The listing builds one solid part. Answer for the finished solid, in the listing's coordinates (mm). A direction names the side the tool comes from. Coordinates: 2 decimals unless noted, no trailing zeros. Write each loop counter-clockwise with the first axis right and the second up, starting at its lowest first coordinate (ties: lowest second). Pieces come first, ordered by that corner, then holes.
(1) Given P1, Ø3.5, axis at x = -12, y = 0.5, coming from the +Z side; P2, Ø12, axis at x = -16, z = 6, coming from the +Y side; P3, Ø0.9, axis at x = -11, y = -1.5, coming from the +Z side; P4, Ø3, axis at x = -17, y = -2, coming from the +Z side, each flat-ended and moving along its own axis, determine where each tip first touches the part or whether it passes through.
(2) The part is cut by section B-B on y = -2.05. Determine the outline of the cut face in (x, z), plus the area to 3 significant figures.
(3) Which of the six approach directions +Z, -Z, +X, -X, +Y, -Y give full straight-line access (tool end or side, diameter ignored) to faces 4 (the flat face through (-13, 0, -10)), 5 (the flat face through (-10.495, -0.042, 11.702)), 6 (the flat face through (-10, 0, -13)), 7 (the cylindrical face through (-0.07, -0.04, -1.5))?
(4) Straight lines are drawn through the part: line 1 (X direction, y = 0.7, z = 0); line 2 (Z direction, x = -8.75, y = 0.3); line 3 (Z direction, x = -12.5, y = 0.7). For each, find the intervals that lie inside material, in ascending order.
(5) The part is cut by section C-C on z = -15. Determine the outline of the cut face in (x, y).
(6) The part is cut by section A-A on z = 0. Determine the outline of the cut face in (x, y), plus the area to 3 significant figures.
(7) For a pull along Z with two mould halves and no side action, classify faces 1 (the flat face through (-12, 0, -11.5)), 2 (the cylindrical face through (-19.43, -0.04, -20.4)), 3 (the cylindrical face through (4, 0, -3)) as +Z half, -Z half, draft (parallel to the pull), parting line (faces both ways), or undercut.
(8) The part is cut by section D-D on x = -2.5. Determine the outline of the cut face in (y, z).
Autodesk Inventor part; units mm, degrees
ref_plane "YZ Plane" through (0, 0, 0) normal (1, 0, 0) x (0, 1, 0)
ref_plane "XZ Plane" through (0, 0, 0) normal (0, 1, 0) x (-1, 0, 0)
ref_plane "XY Plane" through (0, 0, 0) normal (0, 0, 1) x (1, 0, 0)
sketch "Szkic1" plane through (0, 0, 0) normal (0, 1, 0) x (-1, 0, 0)
  arc A0 (13.307, 18.2188) -> (4.1253, 22.1807) centre (8.7161, 20.1997) ccw
  line L0 (4.1253, 22.1807) -> (-4.5909, 1.9809)
  line L1 (13.307, 18.2188) -> (7.6031, 5)
  arc A1 (-4.5909, 1.9809) -> (0, -5) centre (0, 0) ccw
  line L2 (8, -5) -> (10.5, -5) construction
  line L3 (10, -19) -> (10, -20)
  line L4 (10, -20) -> (10, -21)
  line L5 (10, -7) -> (10, -5)
  line L6 (10, -12) -> (10, -14)
  line L7 (10, -14) -> (10, -14.5)
  line L8 (20, -21) -> (10, -21)
  line L9 (13, -18) -> (10, -18)
  line L10 (10, -18) -> (10, -19)
  line L11 (10, -7) -> (10, -8)
  line L12 (10, -8) -> (13, -8)
  line L13 (13, -11.5) -> (10, -11.5)
  line L14 (10, -11.5) -> (10, -12)
  line L15 (13, -14.5) -> (10, -14.5)
  line L16 (10, -18) -> (13, -18)
  line L17 (13, -8) -> (13, -11.5)
  line L18 (13, -14.5) -> (13, -18)
  line L19 (18, 5) -> (20, 5)
  line L20 (20, 5) -> (20, -21)
  line L21 (20, -21) -> (18, -21)
  line L22 (0, -5) -> (10, -5)
  line L23 (18, 5) -> (7.6031, 5)
  arc A2 (13.307, 18.2188) -> (4.1253, 22.1807) centre (8.7161, 20.1997) ccw
extrude "Wyciągnięcie proste6" add sketch "Szkic1" along normal mid plane 6
fillet "Zaokrąglenie3" radius 2 2 edges at (-20, 0, -21) (-20, 0, 5)
fillet_without_effect "Fillet4"
sketch "Sketch8" plane through (0, 3, 0) normal (0, 1, 0) x (1, 0, 0)
  point P0 (0, 0)
  point P1 (0, 0)
hole "Hole1" at (0, 3, 0) direction (0, -1, 0) diameter 3 end through all
sketch "Sketch9" plane through (0, 3, 0) normal (0, 1, 0) x (1, 0, 0)
  arc A0 (-13.307, -18.2188) -> (-4.1253, -22.1807) centre (-8.7161, -20.1997) ccw
  point P0 (0, 0)
hole "Hole2" at (-8.7161, 3, 20.1997) direction (0, -1, 0) diameter 3 end through all
properties part number "Chwytak wersja 3 - baza"
Model answer:
1. P1: stops at z = 24.96
1. P2: stops at y = 3
1. P3: stops at z = 24.85
1. P4: stops at z = 5
2. outline: (-20, -19) arc R2 ccw to (-18, -21) - (-10, -21) - (-10, -18) - (-13, -18) - (-13, -14.5) - (-10, -14.5) - (-10, -11.5) - (-13, -11.5) - (-13, -8) - (-10, -8) - (-10, -5) - (0, -5) arc R5 ccw to (4.59, 1.98) - (-4.13, 22.18) arc R5 ccw to (-13.31, 18.22) - (-7.6, 5) - (-18, 5) arc R2 ccw to (-20, 3) - close; hole circle Ø3 at (-8.72, 20.2); hole circle Ø3 at (0, 0)
2. area: 569 mm2
3. face 4: +X, +Y, -Y
3. face 5: -X, +Y, -Y
3. face 6: -Z, +X, +Y, -Y
3. face 7: +Y, -Y
4. line 1: x = -20 to -1.5, 1.5 to 5
4. line 2: z = -5 to 5, 7.66 to 18.7, 21.7 to 25.2
4. line 3: z = -21 to -18, -14.5 to -11.5, -8 to 5, 16.35 to 23.47
5. outline: (-20, -3) - (-13, -3) - (-13, 3) - (-20, 3) - close
6. outline: (-20, -3) - (-1.5, -3) - (-1.5, 3) - (-20, 3) - close; (1.5, -3) - (5, -3) - (5, 3) - (1.5, 3) - close
6. area: 132 mm2
7. face 1: undercut
7. face 2: -Z half
7. face 3: parting line
8. outline: (-3, -5) - (3, -5) - (3, 18.41) - (-3, 18.41) - close
